from build123d import *

# Parameters (mm, degrees)
F0_R     = 100
F0_R_2   = 25
F1_DEPTH = 32.5
F2_T     = -5


with BuildPart() as f1:
    # F0 (on Front) → F1 (new body, symmetric)
    with BuildSketch(Plane.XZ):
        Circle(F0_R)
        Circle(F0_R_2, mode=Mode.SUBTRACT)
    extrude(amount=F1_DEPTH, both=True)

    # F2
    f2_openings = [f1.faces().sort_by_distance(p)[0] for p in [
        (-100, 0, 0),
    ]]
    offset(amount=F2_T, openings=f2_openings)


solid = f1.part
For this review, take the finished solid that the model builds, in its own axes (mm). A direction names the side the tool comes from. Give positions to 0.01 mm unless a question says otherwise; leave off trailing zeros. Order: outer loops, then holes, each group sorted by start corner. A loop starts at its lowest first (then second) coordinate and runs counter-clockwise, first axis right, second up. Notation, with made-up numbers: (70.25, 16.5) - (79.25, 16.5) arc R19 ccw to (79.25, 52.5) - close; hole circle Ø6 at (-32, -25). An arc over 180 degrees is marked (long way). Answer as a JSON object with one key per item and string values. Group by question number.
Item 1: Clearance check with flat-ended pins moving along their axes: pin 1 Ø4 at (y, z) = (5.5, 26.5) entering from +X; pin 2 Ø5 at (y, z) = (-7, 33.5) entering from -X; pin 3 Ø10 at (y, z) = (-11, -25) entering from -X; pin 4 Ø1 at (y, z) = (-13, -9.5) entering from -X. State where each tip first meets the part, or that it passes through.
Item 2: Draft analysis for pull direction X (two halves, no side actions). For faces 3 (the cylindrical face through (95.38, 29.96, 30.04)), 4 (the cylindrical face through (23.846, 0.455, 7.509)), 5 (the flat face through (21, -32.5, -21)), state which applies: pulls with the +X half, pulls with the -X half, needs draft (parallel to the pull), parting line crosses it, or undercut.
Item 3: Wall thickness on line 1 along Z through (x, y) = (0, 7); line 2 along Y through (x, z) = (-1.5, -64.5); line 3 along X through (y, z) = (6, 14): over which ranges is each line inside the solid? List them lowest first.
Item 4: Take a section at D-D on z = -44. Give the boundary of the cut face in (x, y).
Item 5: Take a section at C-C on x = -51. Give the boundary of the cut face in (y, z).
Item 6: Take a section at A-A on z = 0. Give the boundary of the cut face in (x, y), and give its area (3 significant figures).
Item 7: Machinability: for faces 1 (the cylindrical face through (95.38, -30.04, 30.04)), 2 (the cylindrical face through (-29.97, 0.39, 1.32)), which of the approach directions +Z, -Z, +X, -X, +Y, -Y give a long, thin tool a straight path to every point of the face, cutting with its end or side? Answer none if there is none.
Item 8: Take a section at B-B on x = 0. Give the boundary of the cut face in (y, z).
Reported:
{
 "1": {"pin 1": "x = 17.31", "pin 2": "through", "pin 3": "x = -22.36", "pin 4": "x = -28.62"},
 "2": {"face 3": "parting line crosses it", "face 4": "undercut", "face 5": "needs draft"},
 "3": {"line 1": "-30 to -25, 25 to 30", "line 2": "-32.5 to -27.5, 27.5 to 32.5", "line 3": "-26.53 to -20.71, 20.71 to 26.53"},
 "4": {"outline": "(-89.8, -32.5) - (89.8, -32.5) - (89.8, -27.5) - (-89.8, -27.5) - close; (-89.8, 27.5) - (89.8, 27.5) - (89.8, 32.5) - (-89.8, 32.5) - close"},
 "5": {"outline": "(-32.5, -86.02) - (-27.5, -86.02) - (-27.5, 86.02) - (-32.5, 86.02) - close; (27.5, -86.02) - (32.5, -86.02) - (32.5, 86.02) - (27.5, 86.02) - close"},
 "6": {"outline": "(-100, -32.5) - (-25, -32.5) - (-25, 32.5) - (-100, 32.5) - (-100, 27.5) - (-30, 27.5) - (-30, -27.5) - (-100, -27.5) - close; (25, -32.5) - (100, -32.5) - (100, -27.5) - (30, -27.5) - (30, 27.5) - (100, 27.5) - (100, 32.5) - (25, 32.5) - close", "area": "2,050 mm^2"},
 "7": {"face 1": "+Y, -Y", "face 2": "none"},
 "8": {"outline": "(-32.5, -100) - (-27.5, -100) - (-27.5, -30) - (27.5, -30) - (27.5, -100) - (32.5, -100) - (32.5, -25) - (-32.5, -25) - close; (-32.5, 25) - (32.5, 25) - (32.5, 100) - (27.5, 100) - (27.5, 30) - (-27.5, 30) - (-27.5, 100) - (-32.5, 100) - close"}
}
